```python
from build123d import *

# Parameters (mm, degrees)
F0_W     = 16.9418
F0_H     = 100.0506
F1_DEPTH = 2.54


with BuildPart() as f1:
    # F0 (on Front) → F1 (new body)
    with BuildSketch(Plane.XZ):
        Polygon((-12.7, 0), (0, 0), (12.7, 0), (12.7, 34.9758), (10.469878, 34.9758), (-10.469878, 34.9758), (-12.7, 34.9758), align=None)
        Polygon((-10.469878, 85.0138), (-10.469878, 34.9758), (10.469878, 34.9758), (10.469878, 85.0138), (8.4709, 85.0138), (-8.4709, 85.0138), align=None)
        with Locations((0, 135.0391)):
            Rectangle(F0_W, F0_H)
    extrude(amount=-F1_DEPTH)


solid = f1.part
```
Geometry check sheet. Reference: the model listing, model coordinates, mm. Coordinates: 2 decimals unless noted, no trailing zeros. Loops run counter-clockwise (first coordinate to the right, second up) from the corner with the lowest first, then second, coordinate; pieces in that order, holes last. Notation, with made-up numbers: (71.5, 74.5) -> (104.5, 74.5) arc R13 ccw to (104.5, 81.5) -> close; hole circle Ø6 at (-32.75, -6.5). An arc over 180 degrees is marked (long way). Put each result on its own line as item: value.
1) Cross-section at B-B on z = 60. Record the boundary of the cut face in (x, y), plus the area to 3 significant figures.
Result set:
outline: (-10.47, 0) -> (10.47, 0) -> (10.47, 2.54) -> (-10.47, 2.54) -> close
area: 53.2 mm^2
2) Thickness scan on line 1 (Z direction, x = 9.75, y = 1.7); line 2 (Z direction, x = -10.5, y = 0.25); line 3 (X direction, y = 0.45, z = 178.5). Record the ranges inside material, lowest first.
Result set:
line 1: z = 0 to 85.01
line 2: z = 0 to 34.98
line 3: x = -8.47 to 8.47
3) Cross-section at C-C on z = 113.5. Record the boundary of the cut face in (x, y), plus the area to 3 significant figures.
Result set:
outline: (-8.47, 0) -> (8.47, 0) -> (8.47, 2.54) -> (-8.47, 2.54) -> close
area: 43.0 mm^2
4) Gauge pin test, flat ends, axial feed: pin 1 Ø0.8 at (y, z) = (1.5, 157) entering from +X; pin 2 Ø0.8 at (y, z) = (1, 143) entering from -X; pin 3 Ø1.5 at (x, z) = (-2.5, 96) entering from -Y; pin 4 Ø1 at (x, y) = (9.5, 1.5) entering from +Z. Record the tip position at first contact, or that the pin passes through.
Result set:
pin 1: stops at x = 8.47
pin 2: stops at x = -8.47
pin 3: stops at y = 0
pin 4: stops at z = 85.01
5) Cross-section at A-A on y = 1. Record the boundary of the cut face in (x, z), plus the area to 3 significant figures.
Result set:
outline: (-12.7, 0) -> (12.7, 0) -> (12.7, 34.98) -> (10.47, 34.98) -> (10.47, 85.01) -> (8.47, 85.01) -> (8.47, 185.06) -> (-8.47, 185.06) -> (-8.47, 85.01) -> (-10.47, 85.01) -> (-10.47, 34.98) -> (-12.7, 34.98) -> close
area: 3,630 mm^2
